Can you work these out from the model? Positions are in its coordinate system, mm. Face numbers are marked on the shaded views. A direction names the side the tool comes from. Coordinates: 2 decimals unless noted, no trailing zeros. Order: outer loops, then holes, each group sorted by start corner. A loop starts at its lowest first (then second) coordinate and runs counter-clockwise, first axis right, second up. Notation, with made-up numbers: (83, 32) -> (135, 32) arc R28 cw to (135, 71) -> close; hole circle Ø4 at (67.5, -19.75). An arc over 180 degrees is marked (long way). Answer as a JSON object with one key per item and string values. Group by question number.
(1) I want a section at A-A, the plane z = 0. List the corners of the cut face in (x, y) for me.
(2) I need wall thicknesses on line 1 (Y direction, x = -9.5, z = 0); line 2 (Y direction, x = -25, z = 0); line 3 (Z direction, x = -28, y = -18.5). Which ranges of each line are inside material? Lowest first, please.
(3) For pin 1 (5 mm diameter, centred on y = 0.5, z = 5.5, fed in from -X); pin 2 (6 mm diameter, centred on y = -17.5, z = -21.5, fed in from -X); pin 3 (12 mm diameter, centred on x = 53, z = 36, fed in from -Y), each with a flat end and sliding along its axis, tell me the tip position at first contact or that it passes through.
(4) I want a section at C-C, the plane x = -17.5. List the corners of the cut face in (y, z) for me.
(5) Which directions (+Z, -Z, +X, -X, +Y, -Y) give clear straight access to the entire face, cutting with the end or side of a thin tool? Please do the marked faces 4 and 5.
(6) If we mould it in two halves opening along X, with no side actions, what happens to the marked faces 1, 2 and 3? For each: pulls with the +X half, pulls with the -X half, needs draft (parallel to the pull), parting line crosses it, or undercut.
(7) I want a section at B-B, the plane y = 0. List the corners of the cut face in (x, z) for me, plus the area to 3 significant figures.
from build123d import *

# Parameters (mm, degrees)
SKETCH3_R          = 1.778
CUT_EXTRUDE1_DEPTH = 12.7


with BuildPart() as part:
    # Sketch1 → Revolve1 (revolve)
    with BuildSketch(Plane.XY, mode=Mode.PRIVATE) as revolve1_sk:
        Polygon((0, 15.5575), (83.038845842, 63.5), (83.038845842, 57.15), (0, 7.9375), (-12.7, 7.9375), (-33.047266862, 44.45), (-33.047266862, 50.8), (-33.047266862, 63.5), (-20.347266862, 63.5), (-20.347266862, 28.802954744), (-12.7, 15.5575), align=None)
    revolve(revolve1_sk.sketch.rotate(Axis((0, 0, 0), (1, 0, 0)), 90), axis=Axis((0, 0, 0), (1, 0, 0)))

    # Sketch3 → Cut-Extrude1 (cut)
    with BuildSketch(Plane.ZY.offset(33.047266862)):
        with Locations((56.912428742, -5.205569588)):
            Circle(SKETCH3_R)
        with Locations((0, 57.15)):
            Circle(SKETCH3_R)
        with Locations((-57.15, 0)):
            Circle(SKETCH3_R)
        with Locations((-27.61584041, 50.034866428)):
            Circle(SKETCH3_R)
        with Locations((-49.493351826, 28.575)):
            Circle(SKETCH3_R)
        with Locations((28.575, 49.493351826)):
            Circle(SKETCH3_R)
        with Locations((49.682843524, 28.244248253)):
            Circle(SKETCH3_R)
        with Locations((-30.522003084, -48.31697246)):
            Circle(SKETCH3_R)
        with Locations((-50.034866428, -27.61584041)):
            Circle(SKETCH3_R)
        with Locations((46.684824287, -32.964369875)):
            Circle(SKETCH3_R)
        with Locations((28.49967153, -49.536766373)):
            Circle(SKETCH3_R)
        with Locations((0, -57.15)):
            Circle(SKETCH3_R)
    extrude(amount=-CUT_EXTRUDE1_DEPTH, mode=Mode.SUBTRACT)


solid = part.part
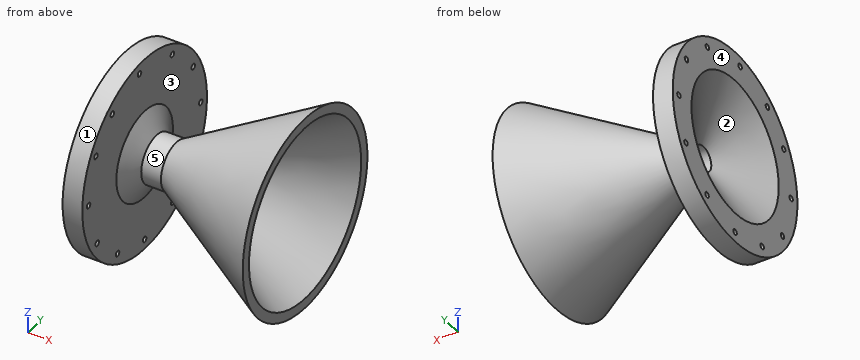
Computed values:
{
 "1": {"outline": "(-33.05, -63.5) -> (-20.35, -63.5) -> (-20.35, -58.93) -> (-33.05, -58.93) -> close; (-33.05, -55.37) -> (-20.35, -55.37) -> (-20.35, -28.8) -> (-12.7, -15.56) -> (0, -15.56) -> (83.04, -63.5) -> (83.04, -57.15) -> (0, -7.94) -> (-12.7, -7.94) -> (-33.05, -44.45) -> close; (-33.05, 44.45) -> (-12.7, 7.94) -> (0, 7.94) -> (83.04, 57.15) -> (83.04, 63.5) -> (0, 15.56) -> (-12.7, 15.56) -> (-20.35, 28.8) -> (-20.35, 55.37) -> (-33.05, 55.37) -> close; (-33.05, 58.93) -> (-20.35, 58.93) -> (-20.35, 63.5) -> (-33.05, 63.5) -> close"},
 "2": {"line 1": "y = -15.56 to -7.94, 7.94 to 15.56", "line 2": "y = -63.5 to -58.93, -55.37 to -30.01, 30.01 to 55.37, 58.93 to 63.5", "line 3": "z = -60.75 to -30.17, 30.17 to 60.75"},
 "3": {"pin 1": "stops at x = -12.75", "pin 2": "stops at x = -25.4", "pin 3": "stops at y = -36.81"},
 "4": {"outline": "circle Ø47.74 at (0, 0); hole circle Ø33.1 at (0, 0)"},
 "5": {"face 4": "+Z, -Z, -X, +Y, -Y", "face 5": "none"},
 "6": {"face 1": "needs draft", "face 2": "pulls with the -X half", "face 3": "undercut"},
 "7": {"outline": "(-33.05, -63.5) -> (-20.35, -63.5) -> (-20.35, -58.93) -> (-33.05, -58.93) -> close; (-33.05, -55.37) -> (-20.35, -55.37) -> (-20.35, -28.8) -> (-12.7, -15.56) -> (0, -15.56) -> (83.04, -63.5) -> (83.04, -57.15) -> (0, -7.94) -> (-12.7, -7.94) -> (-33.05, -44.45) -> close; (-33.05, 44.45) -> (-12.7, 7.94) -> (0, 7.94) -> (83.04, 57.15) -> (83.04, 63.5) -> (0, 15.56) -> (-12.7, 15.56) -> (-20.35, 28.8) -> (-20.35, 63.5) -> (-33.05, 63.5) -> close", "area": "2,190 mm2"}
}
